```python
from build123d import *

# Parameters (mm, degrees)
F0_R          = 9.525
F1_DEPTH      = 127
F2_R          = 9.525
F3_DEPTH      = 24.892
F3_DEPTH_BACK = 62.992


with BuildPart() as f1:
    # F0 (on Front) → F1 (new body)
    with BuildSketch(Plane.XZ):
        Polygon((6.620656, 42.305574), (-31.479344, 42.305574), (-31.479344, -8.494426), (-21.954344, -8.494426), (-21.954344, -21.194426), (-2.904344, -21.194426), (-2.904344, -8.494426), (6.620656, -8.494426), align=None)
        with Locations((-12.429344, 16.905574)):
            Circle(F0_R, mode=Mode.SUBTRACT)
    extrude(amount=F1_DEPTH)

    # F2 (on Right) → F3 (cut, two sides)
    with BuildSketch(Plane.YZ) as f3_sk:
        with Locations((-31.75, 17.925737)):
            Circle(F2_R)
        with Locations((-95.083454, 17.925737)):
            Circle(F2_R)
    extrude(amount=F3_DEPTH, mode=Mode.SUBTRACT)
    extrude(f3_sk.sketch, amount=-F3_DEPTH_BACK, mode=Mode.SUBTRACT)


solid = f1.part
```
The listing builds one solid part. Answer for the finished solid, in the listing's coordinates (mm). A direction names the side the tool comes from. Give positions to 0.01 mm unless a question says otherwise; leave off trailing zeros. Order: outer loops, then holes, each group sorted by start corner. A loop starts at its lowest first (then second) coordinate and runs counter-clockwise, first axis right, second up. Notation, with made-up numbers: (-32, 43.5) -> (7, 43.5) arc R25 ccw to (7, 76.5) -> close; hole circle Ø5 at (64.5, 50.25). An arc over 180 degrees is marked (long way). Answer as a JSON object with one key per item and string values. Group by question number.
Item 1: A tool of negligible diameter and unlimited length cuts with its end or side. For faces 4 (the flat face through (-21.954, -63, -15)), 5 (the flat face through (-2.904, -63, -15)), 6 (the flat face through (6.621, -63, 17)), from which of +Z, -Z, +X, -X, +Y, -Y can it reach the whole face along a straight path? Write none if from no direction.
Item 2: The part is cut by section B-B on z = 21. Write down the section's boundary in (x, y), and give its area (3 significant figures).
Item 3: Determine the mould class of faces 1 (the flat face through (-12, -63, 42.306)), 2 (the flat face through (-13, -63, -21.194)), 3 (the cylindrical face through (-8.034, -62.611, 8.455)) for opening direction Z: pulls with the +Z half, pulls with the -Z half, needs draft (parallel to the pull), parting line crosses it, or undercut.
Item 4: The part is cut by section D-D on y = -112.5. Write down the section's boundary in (x, z) (3 decimals), and give its area (3 significant figures).
Item 5: Flat-ended cylindrical pins translate along their axes: pin 1 (17 mm diameter, centred on y = -95.08, z = 17.93, fed in from +X); pin 2 (7.5 mm diameter, centred on x = 2.5, y = -88, fed in from -Z); pin 3 (10 mm diameter, centred on y = -57, z = -16, fed in from -X). Find the tip coordinate at first contact, or state that the pin passes through.
Item 6: Consider L1, parallel to Z at x = -13, y = -14; L2, parallel to Z at x = -25.5, y = -114; L3, parallel to Y at x = -6, z = 26. Determine where each line is inside the solid, lowest interval first. Write a range as from..to.
Item 7: The part is cut by section C-C on y = -31.75. Write down the section's boundary in (x, z) (3 decimals).
Item 8: The part is cut by section A-A on x = -16. Write down the section's boundary in (y, z) (3 decimals).
Result set:
{
 "1": {"face 4": "-Z, -X, +Y, -Y", "face 5": "-Z, +X, +Y, -Y", "face 6": "+Z, -Z, +X, +Y, -Y"},
 "2": {"outline": "(-31.48, -127) -> (-21.03, -127) -> (-21.03, -104.1) -> (-31.48, -104.1) -> close; (-31.48, -86.07) -> (-21.03, -86.07) -> (-21.03, -40.77) -> (-31.48, -40.77) -> close; (-31.48, -22.73) -> (-21.03, -22.73) -> (-21.03, 0) -> (-31.48, 0) -> close; (-3.83, -127) -> (6.62, -127) -> (6.62, -104.1) -> (-3.83, -104.1) -> close; (-3.83, -86.07) -> (6.62, -86.07) -> (6.62, -40.77) -> (-3.83, -40.77) -> close; (-3.83, -22.73) -> (6.62, -22.73) -> (6.62, 0) -> (-3.83, 0) -> close", "area": "1,900 mm²"},
 "3": {"face 1": "pulls with the +Z half", "face 2": "pulls with the -Z half", "face 3": "undercut"},
 "4": {"outline": "(-31.479, -8.494) -> (-21.954, -8.494) -> (-21.954, -21.194) -> (-2.904, -21.194) -> (-2.904, -8.494) -> (6.621, -8.494) -> (6.621, 42.306) -> (-31.479, 42.306) -> close; hole circle Ø19.05 at (-12.429, 16.906)", "area": "1,890 mm²"},
 "5": {"pin 1": "through", "pin 2": "z = -8.49", "pin 3": "x = -21.95"},
 "6": {"L1": "-21.19..7.4, 26.41..42.31", "L2": "-8.49..42.31", "L3": "-127..-100.14, -90.03..-36.8, -26.7..0"},
 "7": {"outline": "(-31.479, -8.494) -> (-21.954, -8.494) -> (-21.954, -21.194) -> (-2.904, -21.194) -> (-2.904, -8.494) -> (6.621, -8.494) -> (6.621, 8.401) -> (-8.141, 8.401) arc R9.525 cw to (-16.718, 8.401) -> (-31.479, 8.401) -> close; (-31.479, 27.451) -> (6.621, 27.451) -> (6.621, 42.306) -> (-31.479, 42.306) -> close"},
 "8": {"outline": "(-127, -21.194) -> (0, -21.194) -> (0, 8.075) -> (-127, 8.075) -> close; (-127, 25.736) -> (-100.536, 25.736) arc R9.525 cw to (-89.631, 25.736) -> (-37.202, 25.736) arc R9.525 cw to (-26.298, 25.736) -> (0, 25.736) -> (0, 42.306) -> (-127, 42.306) -> close"}
}
